The listing builds one solid part. Answer for the finished solid, in the listing's coordinates (mm). Round coordinates to 2 decimals unless told otherwise and drop trailing zeros. Order: outer loops, then holes, each group sorted by start corner. A loop starts at its lowest first (then second) coordinate and runs counter-clockwise, first axis right, second up. Notation, with made-up numbers: (16, 56) - (64, 56) arc R24 ccw to (64, 80) - close; hole circle Ø10 at (-8, 80). An arc over 180 degrees is marked (long way). Use CSV: the item, a comma, the result in double quotes. Start each with the question number.
Item 1: A flat-ended cylindrical pin translates along its axis: P1, Ø6, axis at x = -175, y = -55.5, coming from the -Z side. Find the tip coordinate at first contact, or state that the pin passes through.
Item 2: Find section C-C, the plane z = 2.3. Give the vertices of the cut face in (x, y), plus the area to 3 significant figures.
Item 3: Find section B-B, the plane x = -10.16. Give the vertices of the cut face in (y, z) (3 decimals), plus the area to 3 significant figures.
Item 4: Find section D-D, the plane x = -152.4. Give the vertices of the cut face in (y, z) (3 decimals).
Item 5: Find section A-A, the plane x = -294.64. Give the vertices of the cut face in (y, z) (3 decimals), plus the area to 3 significant figures.
Item 6: Straight lines are drawn through the part: line 1 along Y through (x, z) = (-152.4, 1.45); line 2 along Y through (x, z) = (-294.64, 1.9); line 3 along X through (y, z) = (-7.5, 0.35). For each, find the intervals that lie inside material, in ascending order. Write a range as [from, to].
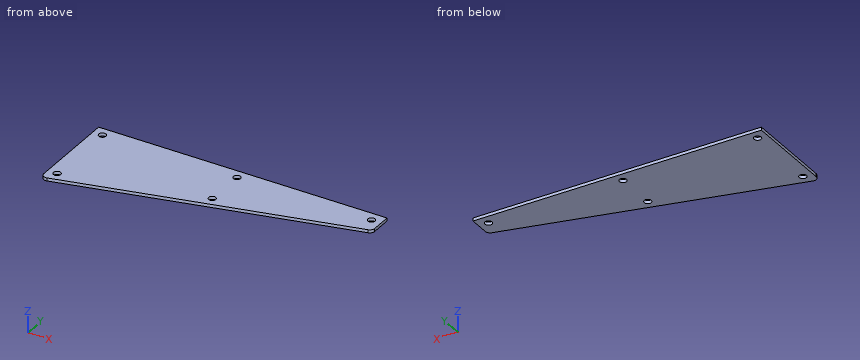
```python
from build123d import *

# Parameters (mm, degrees)
F1_DEPTH = 3.175
F2_R     = 3.81
F3_DEPTH = 25.4


with BuildPart() as f1:
    # F0 (on Top) → F1 (new body)
    with BuildSketch(Plane.XY):
        with BuildLine():
            Line((0, -21.433656), (0, 0))
            Line((0, 0), (-304.8, 0))
            Line((-304.8, 0), (-304.8, -95.093656))
            ThreePointArc((-304.8, -95.093656), (-302.846294, -99.097739), (-298.487919, -100.02198))
            Line((-298.487919, -100.02198), (-3.847919, -26.36198))
            ThreePointArc((-3.847919, -26.36198), (-1.075916, -24.55995), (0, -21.433656))
        make_face()
    extrude(amount=F1_DEPTH)

    # F2 (on face) → F3 (cut)
    with BuildSketch(Plane.XY.offset(3.175)):
        with Locations((-294.64, -10.16)):
            Circle(F2_R)
        with Locations((-152.4, -10.16)):
            Circle(F2_R)
        with Locations((-152.4, -53.027312)):
            Circle(F2_R)
        with Locations((-294.64, -88.587312)):
            Circle(F2_R)
        with Locations((-10.16, -10.16)):
            Circle(F2_R)
    extrude(amount=-F3_DEPTH, mode=Mode.SUBTRACT)


solid = f1.part
```
Worked out:
1,P1,"stops at z = 0"
2,outline,"(-304.8, -95.09) arc R5.08 ccw to (-298.49, -100.02) - (-3.85, -26.36) arc R5.08 ccw to (0, -21.43) - (0, 0) - (-304.8, 0) - close; hole circle Ø7.62 at (-294.64, -88.59); hole circle Ø7.62 at (-294.64, -10.16); hole circle Ø7.62 at (-152.4, -53.03); hole circle Ø7.62 at (-152.4, -10.16); hole circle Ø7.62 at (-10.16, -10.16)"
2,area,"19,100 mm²"
3,outline,"(-27.94, 0) - (-13.97, 0) - (-13.97, 3.175) - (-27.94, 3.175) - close; (-6.35, 0) - (0, 0) - (0, 3.175) - (-6.35, 3.175) - close"
3,area,"64.5 mm²"
4,outline,"(-63.5, 0) - (-56.837, 0) - (-56.837, 3.175) - (-63.5, 3.175) - close; (-49.217, 0) - (-13.97, 0) - (-13.97, 3.175) - (-49.217, 3.175) - close; (-6.35, 0) - (0, 0) - (0, 3.175) - (-6.35, 3.175) - close"
5,outline,"(-99.06, 0) - (-92.397, 0) - (-92.397, 3.175) - (-99.06, 3.175) - close; (-84.777, 0) - (-13.97, 0) - (-13.97, 3.175) - (-84.777, 3.175) - close; (-6.35, 0) - (0, 0) - (0, 3.175) - (-6.35, 3.175) - close"
5,area,"266 mm²"
6,line 1,"y = [-63.5, -56.84], [-49.22, -13.97], [-6.35, 0]"
6,line 2,"y = [-99.06, -92.4], [-84.78, -13.97], [-6.35, 0]"
6,line 3,"x = [-304.8, -297.37], [-291.91, -155.13], [-149.67, -12.89], [-7.43, 0]"
